The listing builds one solid part. Answer for the finished solid, in the listing's coordinates (mm). A direction names the side the tool comes from. Give positions to 0.01 mm unless a question says otherwise; leave off trailing zeros. Write each loop counter-clockwise with the first axis right and the second up, starting at its lowest first coordinate (ties: lowest second). Pieces come first, ordered by that corner, then holes.
```python
from build123d import *

# Parameters (mm, degrees)
F0_R     = 11.5
F1_DEPTH = 3
F2_R     = 1.5
F3_R     = 1.49999
F4_R     = 3.875
F5_DEPTH = 4


# Not quite as in the source:
# - a fillet or chamfer is up to 0.001 mm smaller than in the source, because OpenCascade refuses the exact size


with BuildPart() as f1:
    # F0 (on Top) → F1 (new body)
    with BuildSketch(Plane.XY):
        Circle(F0_R)
    extrude(amount=F1_DEPTH)

    # F2
    f2_edges = [f1.edges().sort_by_distance(p)[0] for p in [
        (-11.5, 0, 3),
    ]]
    fillet(f2_edges, radius=F2_R)

    # F3 (radius 1.5 in the source; OpenCascade refuses exactly that, so slightly less here)
    f3_edges = [f1.edges().sort_by_distance(p)[0] for p in [
        (-11.5, 0, 0),
    ]]
    fillet(f3_edges, radius=F3_R)

    # F4 (on face) → F5 (join)
    with BuildSketch(Plane(origin=(0, 0, 0), x_dir=(1, 0, 0), z_dir=(0, 0, -1))):
        Circle(F4_R)
    extrude(amount=F5_DEPTH)


solid = f1.part
```
Item 1: Consider probe 1 along Z at (x, y) = (-8, -2.5); probe 2 along Y at (x, z) = (4.5, 1); probe 3 along X at (y, z) = (-2.25, -1.25). Determine where each line is inside the solid, lowest interval first.
Conclusion:
probe 1: z = 0 to 3
probe 2: y = -10.49 to 10.49
probe 3: x = -3.15 to 3.15
Item 2: Each of these flat-tipped pins is pushed along its axis until it touches: P1, Ø3, axis at y = 5, z = 0.5, coming from the -X side; P2, Ø1, axis at y = -5, z = 0.5, coming from the +X side; P3, Ø4, axis at y = -1.5, z = 1, coming from the +X side; P4, Ø3, axis at x = -4.5, z = -1, coming from the +Y side. Where does it stop, or does it pass through?
Conclusion:
P1: stops at x = -10.87
P2: stops at x = 10.36
P3: stops at x = 11.5
P4: stops at y = 10.28
Item 3: A cutting plane is placed at C-C, the plane z = -3.5. Give the vertices of the cut face in (x, y) (3 decimals).
Conclusion:
outline: circle Ø7.75 at (0, 0)
Item 4: Which of the six approach directions +Z, -Z, +X, -X, +Y, -Y give full straight-line access (tool end or side, diameter ignored) to faces 1 (the face through (4.3, 0.1, 0)), 2 (the face through (0, 0, -4))?
Conclusion:
face 1: -Z
face 2: -Z, +X, -X, +Y, -Y
